Geometry: final body of the model. Coordinates: model frame, mm. Face numbers are marked on the shaded views. A direction names the side the tool comes from. Give positions to 0.01 mm unless a question says otherwise; leave off trailing zeros. Order: outer loops, then holes, each group sorted by start corner. A loop starts at its lowest first (then second) coordinate and runs counter-clockwise, first axis right, second up. Notation, with made-up numbers: (68, 49.5) -> (124, 49.5) arc R10 ccw to (124, 60.5) -> close; hole circle Ø10 at (-29.75, -27.5). An arc over 180 degrees is marked (long way). One line per question, with ' | ' between items. Start each with the question number.
(1) Ray query, L1, parallel to Z at x = -144.5, y = 17.5; L2, parallel to X at y = 34.5, z = -14.5; L3, parallel to Z at x = -130, y = 28. Return the intervals inside material, ascending.
(2) Section C-C (z = 24). Return loops of the section in (x, y), then the cut area to 3 significant figures.
(3) Set-up query: the marked faces 5 and 6. Return all of +Z, -Z, +X, -X, +Y, -Y with unobstructed straight access to the full face (end or side cutting, diameter ignored); none if empty.
(4) Section A-A (y = 44.5). Return loops of the section in (x, z).
(5) Section B-B (x = -160.5). Return loops of the section in (y, z).
(6) First-contact query: pin 1 Ø4 at (x, z) = (-264.5, -11.5) entering from +Y; pin 2 Ø1 at (y, z) = (41.5, 31) entering from -X; pin 3 Ø4 at (x, z) = (-149, -7.5) entering from +Y; pin 4 Ø1.5 at (x, z) = (-206.5, -9) entering from -Y. Flat tips, straight axial feed; report the tip coordinate or a pass-through.
(7) Mould query, pull axis X, two halves, no side actions, for the marked faces 1, 2, 3 and 4. Classes: +X half, -X half, draft (parallel to the pull), parting line (faces both ways), or undercut.
(8) Section D-D (y = 54). Return loops of the section in (x, z), then the cut area to 3 significant figures.
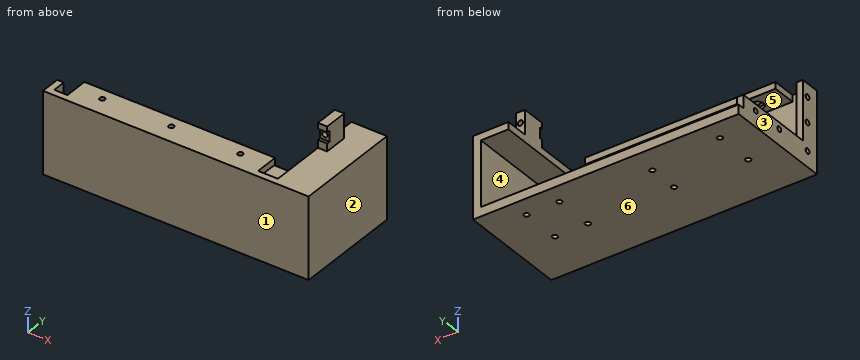
```python
from build123d import *

# Parameters (mm, degrees)
SKETCH1_W           = 182
SKETCH1_H           = 62
BOSS_EXTRUDE1_DEPTH = 5
SKETCH2_W           = 145
SKETCH2_H           = 5
BOSS_EXTRUDE2_DEPTH = 18
SKETCH3_R           = 2
CUT_EXTRUDE1_DEPTH  = 18
SKETCH4_W           = 7
SKETCH4_H           = 62
BOSS_EXTRUDE3_DEPTH = 78
SKETCH5_W           = 175
SKETCH5_H           = 7
BOSS_EXTRUDE4_DEPTH = 78
SKETCH6_W           = 7
SKETCH6_H           = 18
BOSS_EXTRUDE5_DEPTH = 18.5
SKETCH7_R           = 2
CUT_EXTRUDE2_DEPTH  = 18
SKETCH8_W           = 7
SKETCH8_H           = 8.2
CUT_EXTRUDE3_DEPTH  = 2.3
SKETCH9_R           = 4.440846437
SKETCH9_R_2         = 4.5
CUT_EXTRUDE4_DEPTH  = 2.2
SKETCH12_W          = 5
SKETCH12_H          = 55
BOSS_EXTRUDE6_DEPTH = 10
SKETCH13_W          = 5
SKETCH13_H          = 10
BOSS_EXTRUDE7_DEPTH = 63
SKETCH15_R          = 2
CUT_EXTRUDE6_DEPTH  = 63
SKETCH16_W          = 62
SKETCH16_H          = 83
BOSS_EXTRUDE8_DEPTH = 20
SKETCH17_W          = 21
SKETCH17_H          = 49.5
CUT_EXTRUDE7_DEPTH  = 78
SKETCH18_R          = 2
CUT_EXTRUDE8_DEPTH  = 82
SKETCH19_R          = 2
CUT_EXTRUDE9_DEPTH  = 82
SKETCH21_R          = 2
CUT_EXTRUDE10_DEPTH = 10


with BuildPart() as part:
    # Sketch1 → Boss-Extrude1 (new body)
    with BuildSketch(Plane(origin=(0, 0, 0), x_dir=(1, 0, 0), z_dir=(0, 1, 0))):
        with Locations((46.151515152, -7.666666667)):
            Rectangle(SKETCH1_W, SKETCH1_H)
    extrude(amount=BOSS_EXTRUDE1_DEPTH)

    # Sketch2 → Boss-Extrude2 (add)
    with BuildSketch(Plane(origin=(0, 5, 0), x_dir=(1, 0, 0), z_dir=(0, 1, 0))):
        with Locations((49.651515152, -36.166666667)):
            Rectangle(SKETCH2_W, SKETCH2_H)
    extrude(amount=BOSS_EXTRUDE2_DEPTH)

    # Sketch3 → Cut-Extrude1 (cut)
    with BuildSketch(Plane(origin=(0, 0, 33.666666667), x_dir=(-1, 0, 0), z_dir=(0, 0, -1))):
        with Locations((-102.151515152, 14.1)):
            Circle(SKETCH3_R)
        with Locations((-49.651515152, 14.1)):
            Circle(SKETCH3_R)
        with Locations((2.848484848, 14.1)):
            Circle(SKETCH3_R)
    extrude(amount=-CUT_EXTRUDE1_DEPTH, mode=Mode.SUBTRACT)

    # Sketch4 → Boss-Extrude3 (add)
    with BuildSketch(Plane(origin=(0, 5, 0), x_dir=(1, 0, 0), z_dir=(0, 1, 0))):
        with Locations((-41.348484848, -7.666666667)):
            Rectangle(SKETCH4_W, SKETCH4_H)
    extrude(amount=BOSS_EXTRUDE3_DEPTH)

    # Sketch5 → Boss-Extrude4 (add)
    with BuildSketch(Plane(origin=(0, 5, 0), x_dir=(1, 0, 0), z_dir=(0, 1, 0))):
        with Locations((49.651515152, 19.833333333)):
            Rectangle(SKETCH5_W, SKETCH5_H)
    extrude(amount=BOSS_EXTRUDE4_DEPTH)

    # Sketch6 → Boss-Extrude5 (add)
    with BuildSketch(Plane.XY.offset(38.666666667)):
        with Locations((-41.348484848, 56.5)):
            Rectangle(SKETCH6_W, SKETCH6_H)
    extrude(amount=BOSS_EXTRUDE5_DEPTH)

    # Sketch7 → Cut-Extrude2 (cut)
    with BuildSketch(Plane(origin=(0, 65.5, 0), x_dir=(1, 0, 0), z_dir=(0, 1, 0))):
        with Locations((-41.348484848, -48.666666667)):
            Circle(SKETCH7_R)
    extrude(amount=-CUT_EXTRUDE2_DEPTH, mode=Mode.SUBTRACT)

    # Sketch8 → Cut-Extrude3 (cut)
    with BuildSketch(Plane.XZ.offset(-47.5)):
        with Locations((-41.348484848, 48.666666667)):
            Rectangle(SKETCH8_W, SKETCH8_H)
    extrude(amount=-CUT_EXTRUDE3_DEPTH, mode=Mode.SUBTRACT)

    # Sketch9 → Cut-Extrude4 (cut)
    with BuildSketch(Plane(origin=(0, 0, 33.666666667), x_dir=(-1, 0, 0), z_dir=(0, 0, -1))):
        with Locations((-102.151515152, 14.1)):
            Circle(SKETCH9_R)
        with Locations((-49.651515152, 14.1)):
            Circle(SKETCH9_R_2)
        with Locations((2.848484848, 14.1)):
            Circle(SKETCH9_R_2)
    extrude(amount=-CUT_EXTRUDE4_DEPTH, mode=Mode.SUBTRACT)

    # Sketch12 → Boss-Extrude6 (add)
    with BuildSketch(Plane(origin=(0, 5, 0), x_dir=(1, 0, 0), z_dir=(0, 1, 0))):
        with Locations((134.651515152, -11.166666667)):
            Rectangle(SKETCH12_W, SKETCH12_H)
    extrude(amount=BOSS_EXTRUDE6_DEPTH)

    # Sketch13 → Boss-Extrude7 (add)
    with BuildSketch(Plane(origin=(0, 15, 0), x_dir=(1, 0, 0), z_dir=(0, 1, 0))):
        with Locations((134.651515152, 11.333333333)):
            Rectangle(SKETCH13_W, SKETCH13_H)
    extrude(amount=BOSS_EXTRUDE7_DEPTH)

    # Sketch15 → Cut-Extrude6 (cut)
    with BuildSketch(Plane(origin=(137.151515152, 0, 0), x_dir=(0, 0, -1), z_dir=(1, 0, 0))):
        with Locations((11.333333333, 65)):
            Circle(SKETCH15_R)
        with Locations((11.333333333, 40)):
            Circle(SKETCH15_R)
        with Locations((11.333333333, 10)):
            Circle(SKETCH15_R)
        with Locations((-28.666666667, 10)):
            Circle(SKETCH15_R)
        with Locations((-9.666666667, 10)):
            Circle(SKETCH15_R)
    extrude(amount=-CUT_EXTRUDE6_DEPTH, mode=Mode.SUBTRACT)

    # Sketch16 → Boss-Extrude8 (add)
    with BuildSketch(Plane.ZY.offset(44.848484848)):
        with Locations((7.666666667, 41.5)):
            Rectangle(SKETCH16_W, SKETCH16_H)
    extrude(amount=BOSS_EXTRUDE8_DEPTH)

    # Sketch17 → Cut-Extrude7 (cut)
    with BuildSketch(Plane(origin=(0, 83, 0), x_dir=(1, 0, 0), z_dir=(0, 1, 0))):
        with Locations((-48.348484848, -8.416666667)):
            Rectangle(SKETCH17_W, SKETCH17_H)
    extrude(amount=-CUT_EXTRUDE7_DEPTH, mode=Mode.SUBTRACT)

    # Sketch18 → Cut-Extrude8 (cut)
    with BuildSketch(Plane.XY.offset(-16.333333333)):
        with Locations((-34.848484848, 68)):
            Circle(SKETCH18_R)
        with Locations((-9.848484848, 68)):
            Circle(SKETCH18_R)
        with Locations((-34.848484848, 38)):
            Circle(SKETCH18_R)
        with Locations((-9.848484848, 38)):
            Circle(SKETCH18_R)
    extrude(amount=-CUT_EXTRUDE8_DEPTH, mode=Mode.SUBTRACT)

    # Sketch19 → Cut-Extrude9 (cut)
    with BuildSketch(Plane.XY.offset(-16.333333333)):
        with Locations((57.151515152, 63)):
            Circle(SKETCH19_R)
        with Locations((57.151515152, 40)):
            Circle(SKETCH19_R)
    extrude(amount=-CUT_EXTRUDE9_DEPTH, mode=Mode.SUBTRACT)

    # Sketch21 → Cut-Extrude10 (cut)
    with BuildSketch(Plane(origin=(0, 0, -23.333333333), x_dir=(-1, 0, 0), z_dir=(0, 0, -1))):
        with Locations((-112.151515152, 38)):
            Circle(SKETCH21_R)
        with Locations((-112.151515152, 68)):
            Circle(SKETCH21_R)
    extrude(amount=-CUT_EXTRUDE10_DEPTH, mode=Mode.SUBTRACT)


with BuildPart() as body_2:
    # Mirror1: mirrored copy
    add(part.part.mirror(Plane.ZY.offset(64.848484848)))


solid = body_2.part
```
Response:
1) L1: z = -23.33 to -16.33, 33.67 to 38.67 | L2: x = -266.85 to -261.85, -70.85 to -64.85 | L3: z = -23.33 to -16.33
2) outline: (-266.85, 0) -> (-64.85, 0) -> (-64.85, 83) -> (-70.85, 83) -> (-70.85, 5) -> (-261.85, 5) -> (-261.85, 15) -> (-266.85, 15) -> close | area: 1,530 mm^2
3) face 5: +Y | face 6: -Z, +X, -X, +Y, -Y
4) outline: (-266.85, -23.33) -> (-64.85, -23.33) -> (-64.85, 38.67) -> (-91.85, 38.67) -> (-91.85, 33.17) -> (-70.85, 33.17) -> (-70.85, -16.33) -> (-261.85, -16.33) -> (-261.85, -6.33) -> (-266.85, -6.33) -> close
5) outline: (0, -23.33) -> (83, -23.33) -> (83, -16.33) -> (5, -16.33) -> (5, 33.67) -> (23, 33.67) -> (23, 38.67) -> (0, 38.67) -> close
6) pin 1: stops at y = 78 | pin 2: stops at x = -70.85 | pin 3: stops at y = 5 | pin 4: stops at y = 0
7) face 1: draft | face 2: +X half | face 3: -X half | face 4: undercut
8) outline: (-266.85, -23.33) -> (-64.85, -23.33) -> (-64.85, 38.67) -> (-84.85, 38.67) -> (-84.85, 57.17) -> (-91.85, 57.17) -> (-91.85, 33.17) -> (-70.85, 33.17) -> (-70.85, -16.33) -> (-261.85, -16.33) -> (-261.85, -6.33) -> (-266.85, -6.33) -> close; hole circle Ø4 at (-88.35, 48.67) | area: 2,030 mm^2
